For this review, take the finished solid that the model builds, in its own axes (mm). Face numbers are marked on the shaded views. A direction names the side the tool comes from. Round coordinates to 2 decimals unless told otherwise and drop trailing zeros. Loops run counter-clockwise (first coordinate to the right, second up) from the corner with the lowest first, then second, coordinate; pieces in that order, holes last. Notation, with made-up numbers: (77.5, 18.5) -> (121.5, 18.5) arc R25 cw to (121.5, 38.5) -> close; hole circle Ø7 at (-38.5, 34.25). An arc over 180 degrees is marked (long way). Write each question's results on one line, items separated by ' | '.
```python
from build123d import *

# Parameters (mm, degrees)
F1_DEPTH = 25.4
F2_W     = 16.002
F2_H     = 12.954
F3_DEPTH = 25.401
F4_W     = 26.67
F4_H     = 26.67
F5_DEPTH = 22.86
F6_R     = 1.5875
F7_DEPTH = 25.401


with BuildPart() as f1:
    # F0 (on Front) → F1 (new body)
    with BuildSketch(Plane.XZ):
        with BuildLine():
            ThreePointArc((0, -19.05), (14.247427, -9.357442), (21.333408, 6.35))
            ThreePointArc((21.333408, 6.35), (14.960623, 20.045157), (0, 17.959614))
            ThreePointArc((0, 17.959614), (-14.960623, 20.045157), (-21.333408, 6.35))
            ThreePointArc((-21.333408, 6.35), (-14.247427, -9.357442), (0, -19.05))
        make_face()
    extrude(amount=F1_DEPTH)

    # F2 (on face) → F3 (cut, through all)
    with BuildSketch(Plane.XZ.offset(25.4)):
        with Locations((0, 5.207)):
            Rectangle(F2_W, F2_H)
    extrude(amount=-F3_DEPTH, mode=Mode.SUBTRACT)

    # F4 (on face) → F5 (cut)
    with BuildSketch(Plane(origin=(0, 0, 0), x_dir=(-1, 0, 0), z_dir=(0, 1, 0))):
        with Locations((0, 4.318)):
            Rectangle(F4_W, F4_H)
    extrude(amount=-F5_DEPTH, mode=Mode.SUBTRACT)

    # F6 (on face) → F7 (cut, through all)
    with BuildSketch(Plane(origin=(0, 0, 0), x_dir=(-1, 0, 0), z_dir=(0, 1, 0))):
        with Locations((-17.145, 8.89)):
            Circle(F6_R)
        with Locations((17.145, 8.89)):
            Circle(F6_R)
        with Locations((0, -13.97)):
            Circle(F6_R)
    extrude(amount=-F7_DEPTH, mode=Mode.SUBTRACT)


solid = f1.part
```
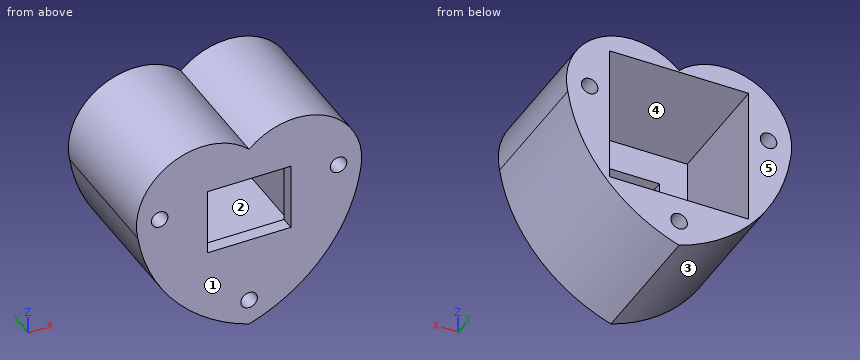
1. Tool access review of the marked faces 4 and 5: name each direction out of +Z, -Z, +X, -X, +Y, -Y from which nothing blocks a thin tool from reaching the whole face with its end or side.
Values found:
face 4: +Y | face 5: +Z, -Z, +X, -X, +Y
2. Consider section B-B (x = -6.5). State the section outline as (y, z) points, plus the area to 3 significant figures.
Values found:
outline: (-25.4, -16.02) -> (0, -16.02) -> (0, -9.02) -> (-22.86, -9.02) -> (-22.86, -1.27) -> (-25.4, -1.27) -> close; (-25.4, 11.68) -> (-22.86, 11.68) -> (-22.86, 17.65) -> (0, 17.65) -> (0, 21.36) -> (-25.4, 21.36) -> close | area: 307 mm2
3. For pin 1 (7 mm diameter, centred on x = 4.5, y = -9, fed in from +Z); pin 2 (2 mm diameter, centred on y = -20.5, z = 2.5, fed in from -X); pin 3 (2 mm diameter, centred on x = 17, y = -8.5, fed in from -Z), all flat-tipped, find the tip position at first contact; note any pin that passes through.
Values found:
pin 1: stops at z = 21.56 | pin 2: stops at x = -20.77 | pin 3: stops at z = -7.07
4. Consider section D-D (y = -5.5). Give the number of separate pieces and of enclosed holes in the cut face, plus the area to 3 significant figures.
Values found:
separate pieces: 1 | enclosed holes: 4 | area: 585 mm2
5. Consider section A-A (z = 8.89). State the section outline as (x, y) points (1 decimal).
Values found:
outline: (-21.6, -25.4) -> (-18.7, -25.4) -> (-18.7, 0) -> (-21.6, 0) -> close; (-15.6, -25.4) -> (-8, -25.4) -> (-8, -22.9) -> (-13.3, -22.9) -> (-13.3, 0) -> (-15.6, 0) -> close; (8, -25.4) -> (15.6, -25.4) -> (15.6, 0) -> (13.3, 0) -> (13.3, -22.9) -> (8, -22.9) -> close; (18.7, -25.4) -> (21.6, -25.4) -> (21.6, 0) -> (18.7, 0) -> close
6. Consider section C-C (z = -13.97). State the section outline as (x, y) points, plus the area to 3 significant figures.
Values found:
outline: (-9.47, -25.4) -> (-1.59, -25.4) -> (-1.59, 0) -> (-9.47, 0) -> close; (1.59, -25.4) -> (9.47, -25.4) -> (9.47, 0) -> (1.59, 0) -> close | area: 400 mm2
7. Draft analysis for pull direction Z (two halves, no side actions). For the marked faces 1, 2 and 3, state which applies: released by +Z, released by -Z, zero draft, split by the parting line, or undercut.
Values found:
face 1: zero draft | face 2: undercut | face 3: released by -Z
8. To check wall thickness, follow probe 1 along Y at (x, z) = (0, 17.5); probe 2 along X at (y, z) = (-9, 20.5); probe 3 along X at (y, z) = (-9.25, 5) (3 decimals). State the ranges of each line that lie inside material, in increasing order.
Values found:
probe 1: y = -25.4 to -22.86 | probe 2: x = -14.04 to -3.74, 3.74 to 14.04 | probe 3: x = -21.101 to -13.335, 13.335 to 21.101
